Autodesk Inventor part; units mm, degrees
ref_plane "YZ Plane" through (0, 0, 0) normal (1, 0, 0) x (0, 1, 0)
ref_plane "XZ Plane" through (0, 0, 0) normal (0, 1, 0) x (-1, 0, 0)
ref_plane "XY Plane" through (0, 0, 0) normal (0, 0, 1) x (1, 0, 0)
sketch "Sketch6" plane through (0, 0, 0) normal (0, 1, 0) x (-1, 0, 0)
  line L0 (356.7, -490) -> (-356.7, -490)
  line L1 (-356.7, -490) -> (-356.7, 490)
  line L2 (-356.7, 490) -> (356.7, 490)
  line L3 (356.7, 490) -> (356.7, -490)
  line L4 (356.7, -490) -> (-356.7, 490) construction
  line L5 (-356.7, -490) -> (356.7, 490) construction
  point P0 (0, 0)
  dimension "d52" = 713.4
  dimension "d53" = 980
extrude "Plate2" add sketch "Sketch6" along normal blind 0.5
sketch "Sketch11" plane through (-356.2, 0, 490) normal (-1, 0, 0) x (0, -1, 0)
  line L0 (0, -980) -> (0, 0)
  line L1 (0, 0) -> (-10, 0)
  line L2 (-10, 0) -> (-10, -980)
  line L3 (-10, -980) -> (0, -980)
edge flange "Flange2" height 10 angle 90 thickness 0.5 bend radius 0.5 thickness toward (-1, 0, 0) relief tear relief width 0.5 relief depth 0.25 edges at (-356.7, 0.5, 0) wall of the first edge with corners at (-356.2, 0, -490) (-356.2, 0, 490) (-356.2, 10, 490) (-356.2, 10, -490)
bend "Bend3"
corner "Corner3"
sketch "Sketch12" plane through (-356.7, 9.5, 490) normal (0, 1, 0) x (-1, 0, 0)
  line L0 (0, -980) -> (0, 0)
  line L1 (0, 0) -> (-10, 0)
  line L2 (-10, 0) -> (-10, -980)
  line L3 (-10, -980) -> (0, -980)
edge flange "Flange3" height 10 angle 90 thickness 0.5 bend radius 0.5 thickness toward (0, 1, 0) relief tear relief width 0.5 relief depth 0.25 edges at (-356.2, 10, 0) wall of the first edge with corners at (-356.7, 9.5, -490) (-356.7, 9.5, 490) (-346.7, 9.5, 490) (-346.7, 9.5, -490)
bend "Bend4"
corner "Corner4"
sketch "Sketch13" plane through (356.2, 0, -490) normal (1, 0, 0) x (0, 1, 0)
  line L0 (0, 980) -> (0, 0)
  line L1 (0, 0) -> (10, 0)
  line L2 (10, 0) -> (10, 980)
  line L3 (10, 980) -> (0, 980)
edge flange "Flange4" height 10 angle 90 thickness 0.5 bend radius 0.5 thickness toward (1, 0, 0) relief tear relief width 0.5 relief depth 0.25 edges at (356.7, 0.5, 0) wall of the first edge with corners at (356.2, 0, 490) (356.2, 0, -490) (356.2, 10, -490) (356.2, 10, 490)
bend "Bend5"
corner "Corner5"
sketch "Sketch14" plane through (356.7, 9.5, -490) normal (0, 1, 0) x (-1, 0, 0)
  line L0 (0, 980) -> (0, 0)
  line L1 (0, 0) -> (10, 0)
  line L2 (10, 0) -> (10, 980)
  line L3 (10, 980) -> (0, 980)
edge flange "Flange5" height 10 angle 90 thickness 0.5 bend radius 0.5 thickness toward (0, 1, 0) relief tear relief width 0.5 relief depth 0.25 edges at (356.2, 10, 0) wall of the first edge with corners at (356.7, 9.5, 490) (356.7, 9.5, -490) (346.7, 9.5, -490) (346.7, 9.5, 490)
bend "Bend6"
corner "Corner6"
equation "\"d52\" = ЖАБРЫ_базовая_ширина - 2 * ЖАБРЫ_шаг_листов"
equation "\"d53\" = ЖАБРЫ_базовая_длина_кор_лист"
equation "\"d54\" = Thickness"
equation "\"d84\" = BendReliefWidth"
equation "\"d85\" = BendReliefDepth"
equation "\"d86\" = MinimumRemnant"
equation "\"d87\" = TransitionRadius"
equation "\"d90\" = BendRadius"
equation "\"d91\" = CornerReliefSize"
equation "\"d92\" = GapSize"
equation "\"d93\" = JacobiRadiusSize"
equation "\"d94\" = BendReliefWidth"
equation "\"d95\" = BendReliefDepth"
equation "\"d96\" = MinimumRemnant"
equation "\"d97\" = TransitionRadius"
equation "\"d100\" = BendRadius"
equation "\"d101\" = CornerReliefSize"
equation "\"d102\" = GapSize"
equation "\"d103\" = JacobiRadiusSize"
equation "\"d104\" = BendReliefWidth"
equation "\"d105\" = BendReliefDepth"
equation "\"d106\" = MinimumRemnant"
equation "\"d107\" = TransitionRadius"
equation "\"d110\" = BendRadius"
equation "\"d111\" = CornerReliefSize"
equation "\"d112\" = GapSize"
equation "\"d113\" = JacobiRadiusSize"
equation "\"d114\" = BendReliefWidth"
equation "\"d115\" = BendReliefDepth"
equation "\"d116\" = MinimumRemnant"
equation "\"d117\" = TransitionRadius"
equation "\"d120\" = BendRadius"
equation "\"d121\" = CornerReliefSize"
equation "\"d122\" = GapSize"
equation "\"d123\" = JacobiRadiusSize"
equation "\"BendRadius\" = Thickness"
equation "\"BendReliefWidth\" = Thickness"
equation "\"BendReliefDepth\" = 0.5 * Thickness"
equation "\"CornerReliefSize\" = 4 * Thickness"
equation "\"MinimumRemnant\" = 2 * Thickness"
equation "\"TransitionRadius\" = BendRadius"
equation "\"JacobiRadiusSize\" = BendRadius"
equation "\"GapSize\" = Thickness"
properties part number "MSC 805 sheet gills" material "Stainless Steel"
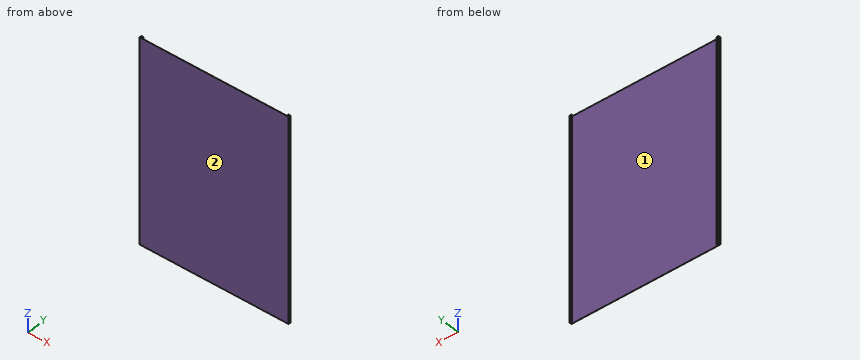
Check sheet for the modelled part. Datum: model origin and axes. Units: mm. Face numbers are marked on the shaded views. Coordinates: 2 decimals unless noted, no trailing zeros. Order: outer loops, then holes, each group sorted by start corner. A loop starts at its lowest first (then second) coordinate and runs counter-clockwise, first axis right, second up. Notation, with made-up numbers: M -4.5,74 L 39.5,74 A31 ccw 39.5,107 Z; hole C 53,76.5 d1. An arc over 180 degrees is marked long. One line per question, with ' | ' between items. Start each with the question number.
Item 1: Mould release check, pull along X, two halves, no side actions. Record for the marked faces 1 and 2: pulls with the +X half, pulls with the -X half, needs draft (parallel to the pull), parting line crosses it, or undercut.
Item 2: Material ranges on line 1 (X direction, y = 4.5, z = 347); line 2 (X direction, y = 0.75, z = 13.5); line 3 (Y direction, x = 327.5, z = 304), recorded low to high.
Item 3: Sectioned sample at C-C on x = -29.5. Record the cut outline in (y, z).
Item 4: Gauge pin test, flat end, axial feed: P1, Ø5, axis at x = -105.5, y = 4, coming from the -Z side. Record the tip position at first contact, or that the pin passes through.
Item 5: Sectioned sample at A-A on y = 5.5. Record the cut outline in (x, z).
Item 6: Sectioned sample at B-B on z = 187. Record the cut outline in (x, y), and give its area (3 significant figures).
Answer below:
1) face 1: undercut | face 2: needs draft
2) line 1: x = -356.7 to -356.2, 356.2 to 356.7 | line 2: x = -356.67 to -356.13, 356.13 to 356.67 | line 3: y = 0 to 0.5
3) outline: M 0,-490 L 0.5,-490 L 0.5,490 L 0,490 Z
4) P1: passes through
5) outline: M -356.7,-490 L -356.2,-490 L -356.2,490 L -356.7,490 Z; M 356.2,-490 L 356.7,-490 L 356.7,490 L 356.2,490 Z
6) outline: M -356.7,1 A1 ccw -355.7,0 L 355.7,0 A1 ccw 356.7,1 L 356.7,9 A1 ccw 355.7,10 L 346.7,10 L 346.7,9.5 L 355.7,9.5 A0.5 cw 356.2,9 L 356.2,1 A0.5 cw 355.7,0.5 L -355.7,0.5 A0.5 cw -356.2,1 L -356.2,9 A0.5 cw -355.7,9.5 L -346.7,9.5 L -346.7,10 L -355.7,10 A1 ccw -356.7,9 Z | area: 375 mm^2
